Answer from the drawing. Dimensions are ordinates in mm from the lowest x, y and z of the part. A direction names the side the tool comes from. Round coordinates to 2 decimals unless told otherwise and drop trailing zeros. Loops run counter-clockwise (first coordinate to the right, second up) from the corner with the lowest first, then second, coordinate; pieces in that order, holes last.
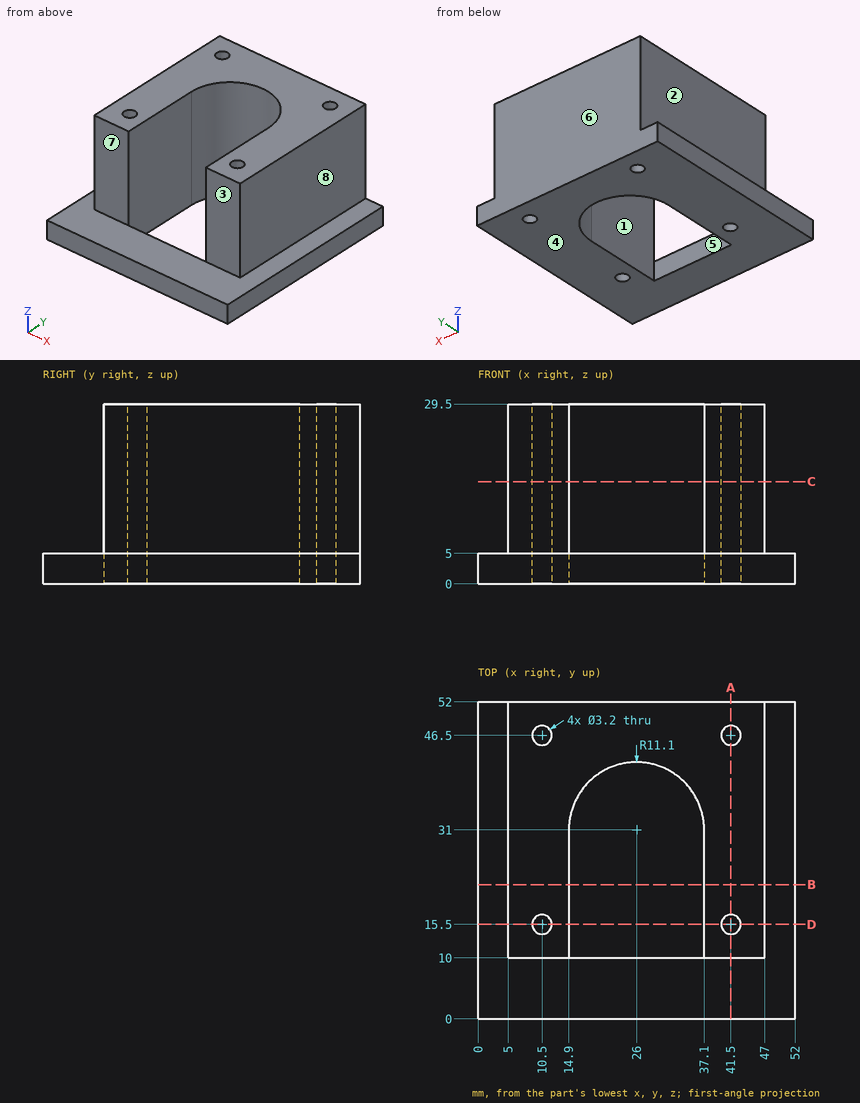
1. Find section A-A (x = 41.5). Write down the section's boundary in (y, z), then the cut area to 3 significant figures.
Answer key:
outline: (0, 0) - (13.9, 0) - (13.9, 29.5) - (10, 29.5) - (10, 5) - (0, 5) - close; (17.1, 0) - (44.9, 0) - (44.9, 29.5) - (17.1, 29.5) - close; (48.1, 0) - (52, 0) - (52, 29.5) - (48.1, 29.5) - close
area: 1,100 mm2
2. Determine the mould class of the marked faces 1, 2 and 3 for opening direction X: +X half, -X half, draft (parallel to the pull), parting line (faces both ways), or undercut.
Answer key:
face 1: undercut
face 2: -X half
face 3: draft
3. Find section C-C (z = 16.75). Write down the section's boundary in (x, y).
Answer key:
outline: (5, 10) - (14.9, 10) - (14.9, 31) arc R11.1 cw to (37.1, 31) - (37.1, 10) - (47, 10) - (47, 52) - (5, 52) - close; hole circle Ø3.2 at (10.5, 15.5); hole circle Ø3.2 at (10.5, 46.5); hole circle Ø3.2 at (41.5, 15.5); hole circle Ø3.2 at (41.5, 46.5)
4. Which of the six approach directions +Z, -Z, +X, -X, +Y, -Y give full straight-line access (tool end or side, diameter ignored) to the marked faces 4, 5, 6, 7 and 8?
Answer key:
face 4: -Z, +X, -X, +Y, -Y
face 5: +Z, -Z
face 6: +Z, -Z, +X, -X, +Y
face 7: +Z, +X, -X, -Y
face 8: +Z, +X, +Y, -Y
5. Find section B-B (y = 22). Write down the section's boundary in (x, z).
Answer key:
outline: (0, 0) - (14.9, 0) - (14.9, 29.5) - (5, 29.5) - (5, 5) - (0, 5) - close; (37.1, 0) - (52, 0) - (52, 5) - (47, 5) - (47, 29.5) - (37.1, 29.5) - close
6. Given pin 1 (10 mm diameter, centred on x = 41.5, y = 45.5, fed in from +Z); pin 2 (6 mm diameter, centred on x = 10, z = 24.5, fed in from -Y); pin 3 (7.5 mm diameter, centred on y = 29.5, z = 19, fed in from -X); pin 4 (17 mm diameter, centred on y = 23, z = 22, fed in from +X), each flat-ended and moving along its own axis, determine where each tip first touches the part or whether it passes through.
Answer key:
pin 1: stops at z = 29.5
pin 2: stops at y = 10
pin 3: stops at x = 5
pin 4: stops at x = 47
7. Consider probe 1 along Y at (x, z) = (41.5, 10); probe 2 along X at (y, z) = (31, 15.5); probe 3 along Z at (x, y) = (50, 12.5). Determine where each line is inside the solid, lowest interval first.
Answer key:
probe 1: y = 10 to 13.9, 17.1 to 44.9, 48.1 to 52
probe 2: x = 5 to 14.9, 37.1 to 47
probe 3: z = 0 to 5
8. Find section D-D (y = 15.5). Write down the section's boundary in (x, z).
Answer key:
outline: (0, 0) - (8.9, 0) - (8.9, 29.5) - (5, 29.5) - (5, 5) - (0, 5) - close; (12.1, 0) - (14.9, 0) - (14.9, 29.5) - (12.1, 29.5) - close; (37.1, 0) - (39.9, 0) - (39.9, 29.5) - (37.1, 29.5) - close; (43.1, 0) - (52, 0) - (52, 5) - (47, 5) - (47, 29.5) - (43.1, 29.5) - close
